Source: CAD feature listing. Evaluate the final solid. Frame: model axes, mm. A direction names the side the tool comes from. Give positions to 0.01 mm unless a question says otherwise; leave off trailing zeros. Order: outer loops, then holes, each group sorted by start corner. A loop starts at its lowest first (then second) coordinate and runs counter-clockwise, first axis right, second up. Notation, with made-up numbers: M 83,20 L 96,20 A35 cw 96,56 Z; hole C 29.5,79 d6. An arc over 180 degrees is marked long. Return JSON: item names as keys, results as strings.
from build123d import *

# Parameters (mm, degrees)
ESQUISSE1_W             = 262
ESQUISSE1_H             = 118.414906094
BOSS_EXTRU_1_DEPTH      = 6
ENL_V_MAT_EXTRU_1_REACH = 281.659
ESQUISSE2_R             = 6.25
ESQUISSE2_W             = 76
ESQUISSE2_H             = 40
ENL_V_MAT_EXTRU_2_REACH = 281.659
ESQUISSE3_R             = 3
ESQUISSE3_R_2           = 1.5
ENL_V_MAT_EXTRU_3_REACH = 281.659
ESQUISSE4_R             = 6.25


with BuildPart() as part:
    # Esquisse1 → Boss.-Extru.1 (new body)
    with BuildSketch(Plane.XY):
        with Locations((-125, -53.207453047)):
            Rectangle(ESQUISSE1_W, ESQUISSE1_H)
    extrude(amount=BOSS_EXTRU_1_DEPTH)

    # Esquisse2 → Enlèv. mat.-Extru.1 (cut, up to next)
    with BuildSketch(Plane.XY.offset(6), mode=Mode.PRIVATE) as enl_v_mat_extru_1_sk1:
        with Locations((-40.5, -23.603726524)):
            Circle(ESQUISSE2_R)
    enl_v_mat_extru_1_tool1 = extrude(enl_v_mat_extru_1_sk1.sketch, amount=-ENL_V_MAT_EXTRU_1_REACH, mode=Mode.PRIVATE) & part.part
    # Esquisse2 → Enlèv. mat.-Extru.1 (cut, up to next)
    with BuildSketch(Plane.XY.offset(6), mode=Mode.PRIVATE) as enl_v_mat_extru_1_sk2:
        with Locations((-78.5, -23.603726524)):
            Circle(ESQUISSE2_R)
    enl_v_mat_extru_1_tool2 = extrude(enl_v_mat_extru_1_sk2.sketch, amount=-ENL_V_MAT_EXTRU_1_REACH, mode=Mode.PRIVATE) & part.part
    # Esquisse2 → Enlèv. mat.-Extru.1 (cut, up to next)
    with BuildSketch(Plane.XY.offset(6), mode=Mode.PRIVATE) as enl_v_mat_extru_1_sk3:
        with Locations((-59.5, -82.811179571)):
            Rectangle(ESQUISSE2_W, ESQUISSE2_H)
    enl_v_mat_extru_1_tool3 = extrude(enl_v_mat_extru_1_sk3.sketch, amount=-ENL_V_MAT_EXTRU_1_REACH, mode=Mode.PRIVATE) & part.part
    add(enl_v_mat_extru_1_tool1.solids().sort_by_distance((-40.5, -23.603727, 6))[0], mode=Mode.SUBTRACT)
    add(enl_v_mat_extru_1_tool2.solids().sort_by_distance((-78.5, -23.603727, 6))[0], mode=Mode.SUBTRACT)
    add(enl_v_mat_extru_1_tool3.solids().sort_by_distance((-59.5, -82.81118, 6))[0], mode=Mode.SUBTRACT)

    # Esquisse3 → Enlèv. mat.-Extru.2 (cut, up to next)
    with BuildSketch(Plane.XY.offset(6), mode=Mode.PRIVATE) as enl_v_mat_extru_2_sk1:
        with Locations((-125, -53.207453047)):
            Circle(ESQUISSE3_R)
    enl_v_mat_extru_2_tool1 = extrude(enl_v_mat_extru_2_sk1.sketch, amount=-ENL_V_MAT_EXTRU_2_REACH, mode=Mode.PRIVATE) & part.part
    # Esquisse3 → Enlèv. mat.-Extru.2 (cut, up to next)
    with BuildSketch(Plane.XY.offset(6), mode=Mode.PRIVATE) as enl_v_mat_extru_2_sk2:
        with Locations((-125, -82.811179571)):
            Circle(ESQUISSE3_R_2)
    enl_v_mat_extru_2_tool2 = extrude(enl_v_mat_extru_2_sk2.sketch, amount=-ENL_V_MAT_EXTRU_2_REACH, mode=Mode.PRIVATE) & part.part
    add(enl_v_mat_extru_2_tool1.solids().sort_by_distance((-125, -53.207453, 6))[0], mode=Mode.SUBTRACT)
    add(enl_v_mat_extru_2_tool2.solids().sort_by_distance((-125, -82.81118, 6))[0], mode=Mode.SUBTRACT)

    # Esquisse4 → Enlèv. mat.-Extru.3 (cut, up to next)
    with BuildSketch(Plane.XY.offset(6), mode=Mode.PRIVATE) as enl_v_mat_extru_3_sk1:
        with Locations((-141.375, -97.613042832)):
            Circle(ESQUISSE4_R)
    enl_v_mat_extru_3_tool1 = extrude(enl_v_mat_extru_3_sk1.sketch, amount=-ENL_V_MAT_EXTRU_3_REACH, mode=Mode.PRIVATE) & part.part
    # Esquisse4 → Enlèv. mat.-Extru.3 (cut, up to next)
    with BuildSketch(Plane.XY.offset(6), mode=Mode.PRIVATE) as enl_v_mat_extru_3_sk2:
        with Locations((-174.125, -97.613042832)):
            Circle(ESQUISSE4_R)
    enl_v_mat_extru_3_tool2 = extrude(enl_v_mat_extru_3_sk2.sketch, amount=-ENL_V_MAT_EXTRU_3_REACH, mode=Mode.PRIVATE) & part.part
    # Esquisse4 → Enlèv. mat.-Extru.3 (cut, up to next)
    with BuildSketch(Plane.XY.offset(6), mode=Mode.PRIVATE) as enl_v_mat_extru_3_sk3:
        with Locations((-206.875, -97.613042832)):
            Circle(ESQUISSE4_R)
    enl_v_mat_extru_3_tool3 = extrude(enl_v_mat_extru_3_sk3.sketch, amount=-ENL_V_MAT_EXTRU_3_REACH, mode=Mode.PRIVATE) & part.part
    # Esquisse4 → Enlèv. mat.-Extru.3 (cut, up to next)
    with BuildSketch(Plane.XY.offset(6), mode=Mode.PRIVATE) as enl_v_mat_extru_3_sk4:
        with Locations((-239.625, -97.613042832)):
            Circle(ESQUISSE4_R)
    enl_v_mat_extru_3_tool4 = extrude(enl_v_mat_extru_3_sk4.sketch, amount=-ENL_V_MAT_EXTRU_3_REACH, mode=Mode.PRIVATE) & part.part
    # Esquisse4 → Enlèv. mat.-Extru.3 (cut, up to next)
    with BuildSketch(Plane.XY.offset(6), mode=Mode.PRIVATE) as enl_v_mat_extru_3_sk5:
        with Locations((-174.125, -68.009316309)):
            Circle(ESQUISSE4_R)
    enl_v_mat_extru_3_tool5 = extrude(enl_v_mat_extru_3_sk5.sketch, amount=-ENL_V_MAT_EXTRU_3_REACH, mode=Mode.PRIVATE) & part.part
    # Esquisse4 → Enlèv. mat.-Extru.3 (cut, up to next)
    with BuildSketch(Plane.XY.offset(6), mode=Mode.PRIVATE) as enl_v_mat_extru_3_sk6:
        with Locations((-206.875, -68.009316309)):
            Circle(ESQUISSE4_R)
    enl_v_mat_extru_3_tool6 = extrude(enl_v_mat_extru_3_sk6.sketch, amount=-ENL_V_MAT_EXTRU_3_REACH, mode=Mode.PRIVATE) & part.part
    # Esquisse4 → Enlèv. mat.-Extru.3 (cut, up to next)
    with BuildSketch(Plane.XY.offset(6), mode=Mode.PRIVATE) as enl_v_mat_extru_3_sk7:
        with Locations((-141.375, -23.603726524)):
            Circle(ESQUISSE4_R)
    enl_v_mat_extru_3_tool7 = extrude(enl_v_mat_extru_3_sk7.sketch, amount=-ENL_V_MAT_EXTRU_3_REACH, mode=Mode.PRIVATE) & part.part
    # Esquisse4 → Enlèv. mat.-Extru.3 (cut, up to next)
    with BuildSketch(Plane.XY.offset(6), mode=Mode.PRIVATE) as enl_v_mat_extru_3_sk8:
        with Locations((-174.125, -23.603726524)):
            Circle(ESQUISSE4_R)
    enl_v_mat_extru_3_tool8 = extrude(enl_v_mat_extru_3_sk8.sketch, amount=-ENL_V_MAT_EXTRU_3_REACH, mode=Mode.PRIVATE) & part.part
    # Esquisse4 → Enlèv. mat.-Extru.3 (cut, up to next)
    with BuildSketch(Plane.XY.offset(6), mode=Mode.PRIVATE) as enl_v_mat_extru_3_sk9:
        with Locations((-206.875, -23.603726524)):
            Circle(ESQUISSE4_R)
    enl_v_mat_extru_3_tool9 = extrude(enl_v_mat_extru_3_sk9.sketch, amount=-ENL_V_MAT_EXTRU_3_REACH, mode=Mode.PRIVATE) & part.part
    # Esquisse4 → Enlèv. mat.-Extru.3 (cut, up to next)
    with BuildSketch(Plane.XY.offset(6), mode=Mode.PRIVATE) as enl_v_mat_extru_3_sk10:
        with Locations((-239.625, -23.603726524)):
            Circle(ESQUISSE4_R)
    enl_v_mat_extru_3_tool10 = extrude(enl_v_mat_extru_3_sk10.sketch, amount=-ENL_V_MAT_EXTRU_3_REACH, mode=Mode.PRIVATE) & part.part
    add(enl_v_mat_extru_3_tool1.solids().sort_by_distance((-141.375, -97.613043, 6))[0], mode=Mode.SUBTRACT)
    add(enl_v_mat_extru_3_tool2.solids().sort_by_distance((-174.125, -97.613043, 6))[0], mode=Mode.SUBTRACT)
    add(enl_v_mat_extru_3_tool3.solids().sort_by_distance((-206.875, -97.613043, 6))[0], mode=Mode.SUBTRACT)
    add(enl_v_mat_extru_3_tool4.solids().sort_by_distance((-239.625, -97.613043, 6))[0], mode=Mode.SUBTRACT)
    add(enl_v_mat_extru_3_tool5.solids().sort_by_distance((-174.125, -68.009316, 6))[0], mode=Mode.SUBTRACT)
    add(enl_v_mat_extru_3_tool6.solids().sort_by_distance((-206.875, -68.009316, 6))[0], mode=Mode.SUBTRACT)
    add(enl_v_mat_extru_3_tool7.solids().sort_by_distance((-141.375, -23.603727, 6))[0], mode=Mode.SUBTRACT)
    add(enl_v_mat_extru_3_tool8.solids().sort_by_distance((-174.125, -23.603727, 6))[0], mode=Mode.SUBTRACT)
    add(enl_v_mat_extru_3_tool9.solids().sort_by_distance((-206.875, -23.603727, 6))[0], mode=Mode.SUBTRACT)
    add(enl_v_mat_extru_3_tool10.solids().sort_by_distance((-239.625, -23.603727, 6))[0], mode=Mode.SUBTRACT)


solid = part.part
1. Set-up query: faces 5 (the face through (-60, -62.811, 3)), 6 (the face through (-127, -112.415, 3)). Return all of +Z, -Z, +X, -X, +Y, -Y with unobstructed straight access to the full face (end or side cutting, diameter ignored); none if empty.
Evaluation:
{"face 5": "+Z, -Z", "face 6": "+Z, -Z, +X, -X, -Y"}
2. Section query C-C (x = -209). Return loops of the section in (y, z), then the cut area to 3 significant figures.
Evaluation:
{"outline": "M -112.41,0 L -103.49,0 L -103.49,6 L -112.41,6 Z; M -91.74,0 L -73.89,0 L -73.89,6 L -91.74,6 Z; M -62.13,0 L -29.48,0 L -29.48,6 L -62.13,6 Z; M -17.73,0 L 6,0 L 6,6 L -17.73,6 Z", "area": "499 mm^2"}
3. Draft query along X for faces 1 (the face through (-135.414, -95.736, 3.042)), 2 (the face through (-21.5, -83, 3)), 3 (the face through (6, -54, 3)), 4 (the face through (-127, -39, 6)). Return one class per face: pulls with the +X half, pulls with the -X half, needs draft (parallel to the pull), parting line crosses it, or undercut.
Evaluation:
{"face 1": "undercut", "face 2": "undercut", "face 3": "pulls with the +X half", "face 4": "needs draft"}
4. Ray query, probe 1 along Y at (x, z) = (-78.5, 1.9); probe 2 along X at (y, z) = (-92, 3.55); probe 3 along Y at (x, z) = (-37, 3.05). Return the intervals inside material, ascending.
Evaluation:
{"probe 1": "y = -112.41 to -102.81, -62.81 to -29.85, -17.35 to 6", "probe 2": "x = -256 to -242.37, -236.88 to -209.62, -204.13 to -176.87, -171.38 to -144.12, -138.63 to -97.5, -21.5 to 6", "probe 3": "y = -112.41 to -102.81, -62.81 to -28.78, -18.43 to 6"}
5. First-contact query: pin 1 (10 mm diameter, centred on x = -78.5, y = -23.6, fed in from +Z). Flat tip, straight axial feed; report the tip coordinate or a pass-through.
Evaluation:
{"pin 1": "passes through"}
6. Section query D-D (z = 1.1). State how many separate pieces and enclosed holes the cut face has, then the cut area to 3 significant figures.
Evaluation:
{"separate pieces": "1", "enclosed holes": "15", "area": "26,500 mm^2"}
7. Section query A-A (y = -78). Return loops of the section in (x, z).
Evaluation:
{"outline": "M -256,0 L -97.5,0 L -97.5,6 L -256,6 Z; M -21.5,0 L 6,0 L 6,6 L -21.5,6 Z"}
8. Section query B-B (x = -40.5). Return loops of the section in (y, z).
Evaluation:
{"outline": "M -112.41,0 L -102.81,0 L -102.81,6 L -112.41,6 Z; M -62.81,0 L -29.85,0 L -29.85,6 L -62.81,6 Z; M -17.35,0 L 6,0 L 6,6 L -17.35,6 Z"}
